Read the model definition and answer for the solid it produces. Units are mm, in the model's axes. A direction names the side the tool comes from. Give positions to 0.01 mm unless a question says otherwise; leave off trailing zeros. Order: outer loops, then holes, each group sorted by start corner. A loop starts at its lowest first (then second) coordinate and runs counter-clockwise, first axis right, second up.
Item 1: A cutting plane is placed at C-C (z = 26). Write down the section's boundary in (x, y) (3 decimals).
Item 2: Which of the six approach directions +Z, -Z, +X, -X, +Y, -Y give full straight-line access (tool end or side, diameter ignored) to faces 3 (the face through (-13, 0, 13)), 4 (the face through (-11.673, 2, -7))?
Item 3: The mould has two halves that part along X. Classify faces 1 (the face through (-13, 2, -4.057)), 2 (the face through (-13, 3.175, 13)): +X half, -X half, draft (parallel to the pull), parting line (faces both ways), or undercut.
Item 4: A cutting plane is placed at B-B (y = 2.15). State how many separate pieces and enclosed holes the cut face has, plus the area to 3 significant figures.
Item 5: A cutting plane is placed at D-D (z = 2). Write down the section's boundary in (x, y) (3 decimals).
Item 6: A cutting plane is placed at A-A (z = -8.5). Write down the section's boundary in (x, y) (3 decimals).
Item 7: Find the intervals of material crossed by line 1 along Z through (x, y) = (-13, 1.8); line 2 along X through (y, z) = (0.85, 42.5); line 3 along Z through (x, y) = (-13.75, 1.6), in increasing order.
Item 8: Given pin 1 Ø1 at (y, z) = (2, -26) entering from -X; pin 2 Ø1 at (x, y) = (-14.5, 2) entering from +Z; pin 3 Ø0.9 at (x, y) = (-13.5, 1) entering from +Z; pin 4 Ø1.6 at (y, z) = (1, -6.5) entering from -X, each flat-ended and moving along its own axis, determine where each tip first touches the part or whether it passes through.
from build123d import *

# Parameters (mm, degrees)
SKETCH1_R           = 1.25
SKETCH1_R_2         = 1.7
SKETCH1_W           = 3.094140016
SKETCH1_H           = 5.373555218
BOSS_EXTRUDE1_DEPTH = 3.175


with BuildPart() as part:
    # Sketch1 → Boss-Extrude1 (new body)
    with BuildSketch(Plane(origin=(0, 0, 0), x_dir=(1, 0, 0), z_dir=(0, 1, 0))):
        with BuildLine():
            Line((-17.941505014, -36.612657571), (-17.206282158, 37.679843625))
            add(Edge.make_bspline(
                [(-17.206282158, 37.679843625), (-17.184484201, 39.873471894), (-15.40321289, 41.64043003), (-13.213298132, 41.640234704)],
                knots=[5, 5, 5, 5, 6, 6, 6, 6], degree=3))
            add(Edge.make_bspline(
                [(-13.213298132, 41.640234704), (-11.02326639, 41.639863585), (-9.242112063, 39.872749187), (-9.220957516, 37.67906232)],
                knots=[6, 6, 6, 6, 7, 7, 7, 7], degree=3))
            Line((-9.220957516, 37.67906232), (-8.499207286, -36.613556071))
            add(Edge.make_bspline(
                [(-8.499207286, -36.613556071), (-8.488347302, -37.73638763), (-8.242642606, -38.944342263), (-7.775936264, -39.965467569)],
                knots=[8, 8, 8, 8, 9, 9, 9, 9], degree=3))
            add(Edge.make_bspline(
                [(-7.775936264, -39.965467569), (-6.625031446, -42.484421072), (-7.34506592, -45.465496377), (-9.518291008, -47.178573835)],
                knots=[0, 0, 0, 0, 1, 1, 1, 1], degree=3))
            add(Edge.make_bspline(
                [(-9.518291008, -47.178573835), (-11.691730567, -48.891651292), (-14.753212643, -48.891270406), (-16.926262256, -47.177802296)],
                knots=[1, 1, 1, 1, 2, 2, 2, 2], degree=3))
            add(Edge.make_bspline(
                [(-16.926262256, -47.177802296), (-19.099292372, -45.464412317), (-19.818819916, -42.483141686), (-18.667408168, -39.96438351)],
                knots=[2, 2, 2, 2, 3, 3, 3, 3], degree=3))
            add(Edge.make_bspline(
                [(-18.667408168, -39.96438351), (-18.200701827, -38.943443763), (-17.952559971, -37.73548913), (-17.941505014, -36.612657571)],
                knots=[3, 3, 3, 3, 4, 4, 4, 4], degree=3))
        make_face()
        with Locations(Location((-13.22099956, -42.362850164, 0), (0, 0, 270))):
            Circle(SKETCH1_R, mode=Mode.SUBTRACT)
        with Locations(Location((-13.213483356, 37.640055716, 0), (0, 0, 270))):
            Circle(SKETCH1_R_2, mode=Mode.SUBTRACT)
        with Locations((-13.219946705, 6.743495147)):
            Rectangle(SKETCH1_W, SKETCH1_H, mode=Mode.SUBTRACT)
    extrude(amount=BOSS_EXTRUDE1_DEPTH)


solid = part.part
Response values:
1. outline: (-17.836, 0) - (-8.602, 0) - (-8.602, 3.175) - (-17.836, 3.175) - close
2. face 3: +Z, -Z, +X, -X, -Y
2. face 4: +Y, -Y
3. face 1: undercut
3. face 2: draft
4. separate pieces: 1
4. enclosed holes: 3
4. area: 760 mm2
5. outline: (-17.599, 0) - (-8.835, 0) - (-8.835, 3.175) - (-17.599, 3.175) - close
6. outline: (-17.495, 0) - (-14.767, 0) - (-14.767, 3.175) - (-17.495, 3.175) - close; (-11.673, 0) - (-8.937, 0) - (-8.937, 3.175) - (-11.673, 3.175) - close
7. line 1: z = -41.63 to -39.33, -35.95 to -9.43, -4.06 to 41.13, 43.59 to 48.46
7. line 2: x = -19.21 to -14.46, -11.98 to -7.23
7. line 3: z = -41.6 to -39.25, -36.03 to -9.43, -4.06 to 41.23, 43.5 to 48.44
8. pin 1: stops at x = -17.33
8. pin 2: stops at z = 48.41
8. pin 3: stops at z = 48.46
8. pin 4: stops at x = -17.52
